Could you check a few things on this model? Use its own coordinates, in mm. A direction names the side the tool comes from. Round coordinates to 2 decimals unless told otherwise and drop trailing zeros. Loops run counter-clockwise (first coordinate to the right, second up) from the corner with the lowest first, then second, coordinate; pieces in that order, holes last. Notation, with made-up numbers: (51, 6.5) -> (66, 6.5) arc R22 ccw to (66, 28.5) -> close; hole circle Ø8 at (56, 4.5). An arc over 180 degrees is marked (long way). One line per item, written item: value.
```python
from build123d import *

# Parameters (mm, degrees)
F0_W     = 38.1
F0_H     = 25.4
F1_DEPTH = 12.7
F3_DEPTH = 38.101
F5_DEPTH = 25.4


with BuildPart() as f1:
    # F0 (on Front) → F1 (new body, symmetric)
    with BuildSketch(Plane.XZ):
        with Locations((19.05, 12.7)):
            Rectangle(F0_W, F0_H)
    extrude(amount=F1_DEPTH, both=True)

    # F2 (on face) → F3 (cut, through all)
    with BuildSketch(Plane.YZ.offset(38.1)):
        Polygon((12.7, 25.4), (-12.7, 25.4), (-12.7, 0), align=None)
    extrude(amount=-F3_DEPTH, mode=Mode.SUBTRACT)

    # F4 (on face) → F5 (cut)
    with BuildSketch(Plane.YZ.offset(38.1)):
        Polygon((0, 0), (0, 12.7), (-12.7, 0), align=None)
    extrude(amount=-F5_DEPTH, mode=Mode.SUBTRACT)


solid = f1.part
```
(1) For pin 1 Ø3 at (x, y) = (4.5, -2.5) entering from +Z; pin 2 Ø5 at (x, y) = (24, 4) entering from +Z; pin 3 Ø4 at (y, z) = (-9, 5) entering from +X, each with a flat end and sliding along its axis, tell me the tip position at first contact or that it passes through.
Results below:
pin 1: stops at z = 11.7
pin 2: stops at z = 19.2
pin 3: stops at x = 12.7
(2) On a 3-axis mill with a long thin cutter (end or side, diameter ignored), from which of +Z, -Z, +X, -X, +Y, -Y can I reach the whole of each face in a straight line? I mean faces 1 (the face through (0, 5, 7)), 2 (the face through (12.7, -4, 4)). Say none if no direction works.
Results below:
face 1: +Z, -Z, -X, +Y, -Y
face 2: +Z, -Z, +X, -Y
(3) Imagine slicing it at A-A on z = 11.5. Write out the boundary of the cut face in (x, y), then the cut area to 3 significant figures.
Results below:
outline: (0, -1.2) -> (12.7, -1.2) -> (12.7, 0) -> (38.1, 0) -> (38.1, 12.7) -> (0, 12.7) -> close
area: 499 mm²
(4) Imagine slicing it at B-B on y = -11. Write out the boundary of the cut face in (x, z).
Results below:
outline: (0, 0) -> (12.7, 0) -> (12.7, 1.7) -> (0, 1.7) -> close
(5) Please list where these lines run through material, in increasing order: L1, parallel to Y at x = 19, z = 4; L2, parallel to Y at x = 17, z = 21.25.
Results below:
L1: y = 0 to 12.7
L2: y = 8.55 to 12.7
(6) Imagine slicing it at C-C on x = 17.5. Write out the boundary of the cut face in (y, z).
Results below:
outline: (0, 0) -> (12.7, 0) -> (12.7, 25.4) -> (0, 12.7) -> close
(7) Imagine slicing it at D-D on z = 4.5. Write out the boundary of the cut face in (x, y), then the cut area to 3 significant figures.
Results below:
outline: (0, -8.2) -> (12.7, -8.2) -> (12.7, 0) -> (38.1, 0) -> (38.1, 12.7) -> (0, 12.7) -> close
area: 588 mm²
